Could you check a few things on this drawing? It's one solid part, dimensions in mm from its lowest x, y, z. Give positions to 0.01 mm unless a question says otherwise; leave off trailing zeros. Loops run counter-clockwise (first coordinate to the right, second up) from the corner with the lowest first, then second, coordinate; pieces in that order, holes last. Notation, with made-up numbers: (-28, 8) - (13, 8) arc R17 cw to (13, 17) - close; hole circle Ø5 at (-35.75, 5). An arc over 180 degrees is marked (long way). Return JSON: item names as keys, results as strings. Group by question number.
(1) If we section it at B-B (y = 3): Please give me the cut outline in (x, z).
(2) If we section it at C-C (z = 34): Please give me the cut outline in (x, y), then the cut area to 3 significant figures.
(3) I need wall thicknesses on probe 1 along Z at (x, y) = (126.5, 52); probe 2 along Y at (x, z) = (38.5, 34.5). Which ranges of each line are inside material? Lowest first, please. Write a range as [from, to].
(4) If we section it at A-A (z = 20): Please give me the cut outline in (x, y), then the cut area to 3 significant figures.
(5) For P1, Ø1.7, axis at x = 5.5, z = 23.5, coming from the +Y side; P2, Ø0.8, axis at y = 2.5, z = 34, coming from the -X side; P3, Ø2, axis at y = 42, z = 22, coming from the -X side, each with a flat end and sliding along its axis, tell me the tip position at first contact or that it passes through.
(6) If we section it at D-D (x = 113): Please give me the cut outline in (y, z).
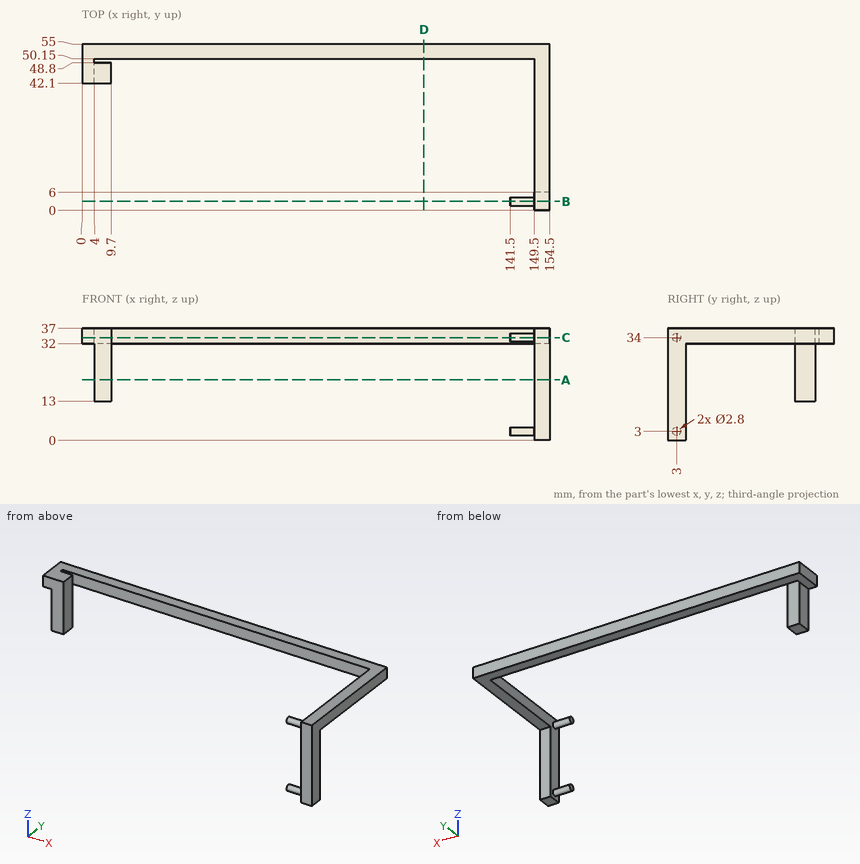
Values:
{
 "1": {"outline": "(141.5, 1.6) - (149.5, 1.6) - (149.5, 0) - (154.5, 0) - (154.5, 37) - (149.5, 37) - (149.5, 35.4) - (141.5, 35.4) - (141.5, 32.6) - (149.5, 32.6) - (149.5, 4.4) - (141.5, 4.4) - close"},
 "2": {"outline": "(0, 42.1) - (9.7, 42.1) - (9.7, 48.8) - (4, 48.8) - (4, 50.15) - (149.5, 50.15) - (149.5, 4.4) - (141.5, 4.4) - (141.5, 1.6) - (149.5, 1.6) - (149.5, 0) - (154.5, 0) - (154.5, 55) - (0, 55) - close", "area": "1,090 mm2"},
 "3": {"probe 1": "[32, 37]", "probe 2": "[50.15, 55]"},
 "4": {"outline": "(4, 42.1) - (9.7, 42.1) - (9.7, 48.8) - (4, 48.8) - close; (149.5, 0) - (154.5, 0) - (154.5, 6) - (149.5, 6) - close", "area": "68.2 mm2"},
 "5": {"P1": "y = 48.8", "P2": "x = 141.5", "P3": "x = 4"},
 "6": {"outline": "(50.15, 32) - (55, 32) - (55, 37) - (50.15, 37) - close"}
}
